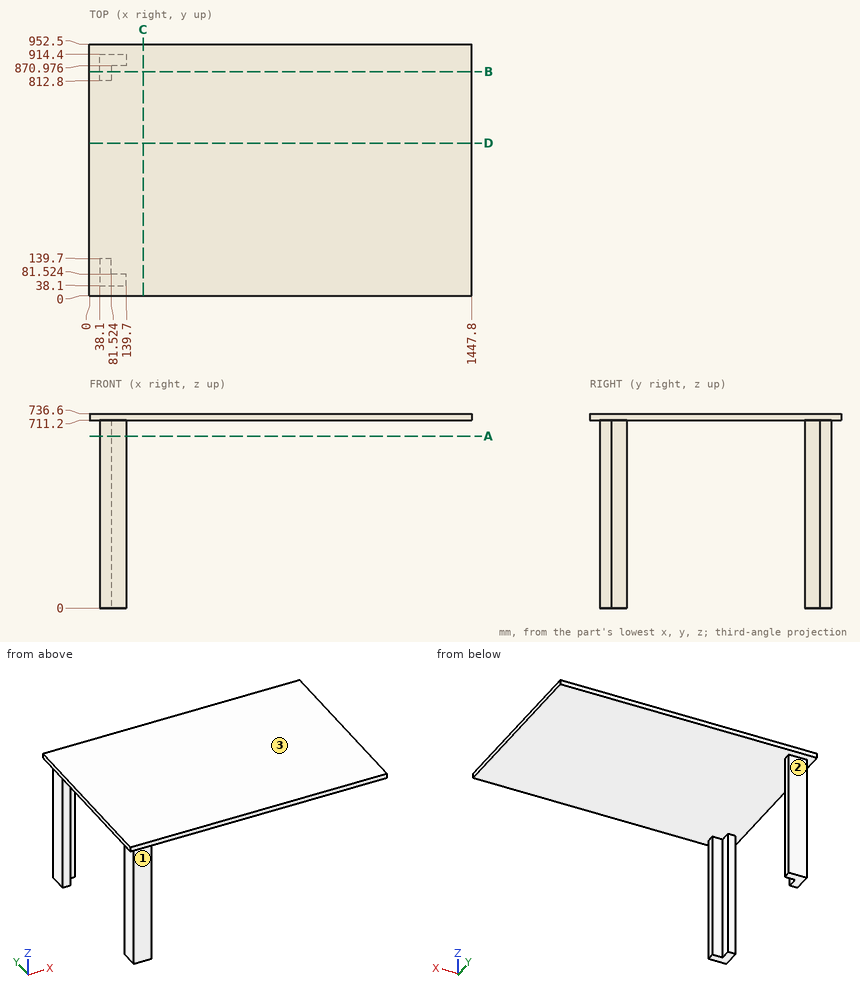
Here's the drawing with two shaded views (mm, measured from the low corner). I have some questions. A direction names the side the tool comes from. Give positions to 0.01 mm unless a question says otherwise; leave off trailing zeros. Write each loop counter-clockwise with the first axis right and the second up, starting at its lowest first coordinate (ties: lowest second). Pieces come first, ordered by that corner, then holes. Notation, with made-up numbers: (-8, -28.5) - (11, -28.5) arc R20 cw to (11, 4.5) - close; hole circle Ø6 at (-11.75, -32.75). An arc over 180 degrees is marked (long way). Write item = value, one per line. Start each with the question number.
1. Please list where these lines run through material, in increasing order: line 1 (Z direction, x = 372.5, y = 289); line 2 (X direction, y = 819, z = 351.5).
2. Imagine slicing it at A-A (z = 651). Please give me the cut outline in (x, y), and give its area (3 significant figures).
3. Imagine slicing it at B-B (y = 847.5). Please give me the cut outline in (x, z), and give its area (3 significant figures).
4. On a 3-axis mill with a long thin cutter (end or side, diameter ignored), from which of +Z, -Z, +X, -X, +Y, -Y can I reach the whole of each face in a straight line? I mean the marked faces 1, 2 and 3. Say none if no direction works.
5. Imagine slicing it at D-D (y = 577). Please give me the cut outline in (x, z), and give its area (3 significant figures).
6. Imagine slicing it at C-C (x = 203). Please give me the cut outline in (y, z).
7. For pin 1 (17.5 mm diameter, centred on x = 119, z = 311, fed in from +Y); pin 2 (17.5 mm diameter, centred on y = 836, z = 278, fed in from +X); pin 3 (21.5 mm diameter, centred on y = 61, z = 532.5, fed in from +X), each with a flat end and sliding along its axis, tell me the tip position at first contact or that it passes through.
Worked answers:
q1.line_1 = 711.2 to 736.6
q1.line_2 = 38.1 to 81.52
q2.outline = (38.1, 38.1) - (139.7, 38.1) - (139.7, 81.52) - (81.52, 81.52) - (81.52, 139.7) - (38.1, 139.7) - close; (38.1, 812.8) - (81.52, 812.8) - (81.52, 870.98) - (139.7, 870.98) - (139.7, 914.4) - (38.1, 914.4) - close
q2.area = 13,900 mm2
q3.outline = (0, 711.2) - (38.1, 711.2) - (38.1, 0) - (81.52, 0) - (81.52, 711.2) - (1447.8, 711.2) - (1447.8, 736.6) - (0, 736.6) - close
q3.area = 67,700 mm2
q4.face_1 = -Z, +X, -X, -Y
q4.face_2 = -Z, +X, -X, +Y
q4.face_3 = +Z, +X, -X, +Y, -Y
q5.outline = (0, 711.2) - (1447.8, 711.2) - (1447.8, 736.6) - (0, 736.6) - close
q5.area = 36,800 mm2
q6.outline = (0, 711.2) - (952.5, 711.2) - (952.5, 736.6) - (0, 736.6) - close
q7.pin_1 = 914.4
q7.pin_2 = 81.52
q7.pin_3 = 139.7
